Part model, mm, in its own coordinate system. A direction names the side the tool comes from. Round coordinates to 2 decimals unless told otherwise and drop trailing zeros. Loops run counter-clockwise (first coordinate to the right, second up) from the corner with the lowest first, then second, coordinate; pieces in that order, holes last. Notation, with made-up numbers: M -38.5,66 L 16.5,66 A26 ccw 16.5,91 Z; hole C 52,76.5 d9. An arc over 180 degrees is marked long. Put each result on its own line as item: value. Start each with the question number.
```python
from build123d import *

# Parameters (mm, degrees)
SKETCH2_R           = 52.5
BOSS_EXTRUDE1_DEPTH = 390
SKETCH3_R           = 30
CUT_EXTRUDE1_DEPTH  = 564.537281534


with BuildPart() as part:
    # Sketch1 → Revolve1 (revolve)
    with BuildSketch(Plane.XY, mode=Mode.PRIVATE) as revolve1_sk:
        Polygon((0, 202.5), (0, -202.5), (75, -202.5), (75, -172.5), (45, -172.5), (45, 202.5), align=None)
    revolve(revolve1_sk.sketch.rotate(Axis((0, 202.5, 0), (0, -1, 0)), 180), axis=Axis((0, 202.5, 0), (0, -1, 0)))

    # Sketch2 → Boss-Extrude1 (add)
    with BuildSketch(Plane(origin=(0, 0, 0), x_dir=(0, 0, 1), z_dir=(0.984807753012208, 0.17364817766693072, 0))):
        with Locations(Location((0, -49.423569985, 0), (0, 0, 31.34866832))):
            Circle(SKETCH2_R)
    extrude(amount=BOSS_EXTRUDE1_DEPTH)

    # Sketch3 → Cut-Extrude1 (cut, through all)
    with BuildSketch(Plane(origin=(0, 202.5, 0), x_dir=(1, 0, 0), z_dir=(0, 1, 0))):
        with Locations(Location((0, 0, 0), (0, 0, 180))):
            Circle(SKETCH3_R)
    extrude(amount=-CUT_EXTRUDE1_DEPTH, mode=Mode.SUBTRACT)


solid = part.part
```
1. Cut at A-A, the plane z = 22. Give the cut face in (x, y).
2. Cut at B-B, the plane y = -38. Give the cut face in (x, z), and give its area (3 significant figures).
3. Drop flat-ended pins along their axis: pin 1 (12 mm diameter, centred on x = 189.5, y = 89.5, fed in from -Z); pin 2 (1 mm diameter, centred on x = 75, y = 16.5, fed in from +Z); pin 3 (12 mm diameter, centred on y = -45, z = -22.5, fed in from +X). Give the stop position or say it passes through.
4. Wall check: L1, parallel to Z at x = 0, y = 5; L2, parallel to Y at x = 60.5, z = -13; L3, parallel to X at y = 172, z = -14. Give the ranges that are in metal, low to high.
5. Which spindle directions (+Z, -Z, +X, -X, +Y, -Y) get a long thin tool onto all of the face, cutting with end or side? Do faces 4 (the flat face through (-8.85, 50.2, -47.66)), 5 (the cylindrical face through (-34.608, -187.29, 66.538)), 6 (the cylindrical face through (-42.92, 17.62, -13.52)). Say none if no direction does.
6. Mould opens along Y. For faces 1 (the flat face through (-1, -202.5, 32)), 2 (the flat face through (-8.785, 49.824, 47.644)), 3 (the flat face through (-9, 202.5, 29)) say: released by +Y, released by -Y, zero draft, split by the parting line, or undercut.
Results list:
1. outline: M -71.7,-202.5 L -20.4,-202.5 L -20.4,202.5 L -39.26,202.5 L -39.26,-172.5 L -71.7,-172.5 Z; M 20.4,-202.5 L 71.7,-202.5 L 71.7,-172.5 L 39.26,-172.5 L 39.26,8.7 L 383.77,69.45 L 367.22,163.34 L 39.26,105.51 L 39.26,202.5 L 20.4,202.5 Z
2. outline: C 0,0 d90; hole C 0,0 d60
2. area: 3,530 mm^2
3. pin 1: stops at z = -52.5
3. pin 2: stops at z = 25.84
3. pin 3: stops at x = 41.87
4. L1: z = -45 to -30, 30 to 45
4. L2: y = -202.5 to -172.5, 9.2 to 112.5
4. L3: x = -42.77 to -26.53, 26.53 to 42.77
5. face 4: -Z, -X
5. face 5: -Y
5. face 6: none
6. face 1: released by -Y
6. face 2: undercut
6. face 3: released by +Y
